Can you work these out from the model? Positions are in its coordinate system, mm. A direction names the side the tool comes from. Round coordinates to 2 decimals unless told otherwise and drop trailing zeros. Write each loop counter-clockwise with the first axis right and the second up, starting at its lowest first coordinate (ties: lowest second). Pieces come first, ordered by that corner, then holes.
Q1. Please list where these lines run through material, in increasing order: line 1 along Z through (x, y) = (-5.5, 0.4); line 2 along X through (y, z) = (1.8, 0); line 3 along Z through (x, y) = (-4, 0.9).
Q2. We'd pull the mould along X, two halves only. Please class faces 1 (the flat face through (0, 0, -1)), 2 (the cylindrical face through (26.99, 1.27, 37.15)), 3 (the flat face through (-13, 1, -20.194)): +X half, -X half, draft (parallel to the pull), parting line (faces both ways), or undercut.
Q3. If we section it at C-C (x = 0): Please give me the cut outline in (y, z).
Q4. If we section it at B-B (z = 3): Please give me the cut outline in (x, y), plus the area to 3 significant figures.
Q5. If we section it at A-A (x = 7): Please give me the cut outline in (y, z), plus the area to 3 significant figures.
Q6. For faces 4 (the flat face through (0, 1, -40)), 5 (the cylindrical face through (0.086, 1.268, -6.983)), which set-ups out of +Z, -Z, +X, -X, +Y, -Y let a thin tool reach every point of the face, with its end or its side?
Q7. If we section it at D-D (y = 0.45): Give the number of separate pieces and of enclosed holes in the cut face, plus the area to 3 significant figures.
from build123d import *

# Parameters (mm, degrees)
SKETCH_1_W          = 60
SKETCH_1_H          = 80
SKETCH_1_R          = 1.25
SKETCH_1_R_2        = 1.6
EXTRUDE_1_DEPTH     = 2.5
FILLET_1_R          = 10
CUT_EXTRUDE_1_DEPTH = 2.5
CUT_EXTRUDE_2_DEPTH = 2.5


with BuildPart() as part:
    # 草图1 → 凸台-拉伸1 (new body)
    with BuildSketch(Plane(origin=(0, 0, 0), x_dir=(1, 0, 0), z_dir=(0, 1, 0))):
        Rectangle(SKETCH_1_W, SKETCH_1_H)
        with Locations(Location((21, 33, 0), (0, 0, 270))):
            Circle(SKETCH_1_R, mode=Mode.SUBTRACT)
        with Locations(Location((-21, 33, 0), (0, 0, 90))):
            Circle(SKETCH_1_R, mode=Mode.SUBTRACT)
        with Locations(Location((-21, -33, 0), (0, 0, 270))):
            Circle(SKETCH_1_R, mode=Mode.SUBTRACT)
        with Locations(Location((21, -33, 0), (0, 0, 90))):
            Circle(SKETCH_1_R, mode=Mode.SUBTRACT)
        with Locations(Location((0, 3, 0), (0, 0, 270))):
            Circle(SKETCH_1_R_2, mode=Mode.SUBTRACT)
        with Locations(Location((3, 0, 0), (0, 0, 270))):
            Circle(SKETCH_1_R_2, mode=Mode.SUBTRACT)
        with Locations(Location((0, -3, 0), (0, 0, 90))):
            Circle(SKETCH_1_R_2, mode=Mode.SUBTRACT)
        with Locations(Location((-3, 0, 0), (0, 0, 90))):
            Circle(SKETCH_1_R_2, mode=Mode.SUBTRACT)
    extrude(amount=EXTRUDE_1_DEPTH)

    # 圆角1
    fillet_1_edges = [part.edges().sort_by_distance(p)[0] for p in [
        (30, 1.25, 40),
        (-30, 1.25, 40),
        (-30, 1.25, -40),
        (30, 1.25, -40),
    ]]
    fillet(fillet_1_edges, radius=FILLET_1_R)

    # 草图2 → 切除-拉伸1 (cut)
    with BuildSketch(Plane(origin=(0, 2.5, 0), x_dir=(1, 0, 0), z_dir=(0, 1, 0))):
        with BuildLine():
            Line((-20.730933361, 20.193862548), (20.730933361, 20.193862548))
            ThreePointArc((20.730933361, 20.193862548), (25.671984835, 15.252811074), (20.730933361, 10.311759599))
            Line((20.730933361, 10.311759599), (-20.730933361, 10.311759599))
            ThreePointArc((-20.730933361, 10.311759599), (-25.671984835, 15.252811074), (-20.730933361, 20.193862548))
        make_face()
        with BuildLine():
            Line((-20.730933361, -20.193862548), (20.730933361, -20.193862548))
            ThreePointArc((20.730933361, -20.193862548), (25.671984835, -15.252811074), (20.730933361, -10.311759599))
            Line((20.730933361, -10.311759599), (-20.730933361, -10.311759599))
            ThreePointArc((-20.730933361, -10.311759599), (-25.671984835, -15.252811074), (-20.730933361, -20.193862548))
        make_face()
    extrude(amount=-CUT_EXTRUDE_1_DEPTH, mode=Mode.SUBTRACT)

    # 草图3 → 切除-拉伸2 (cut)
    with BuildSketch(Plane(origin=(0, 2.5, 0), x_dir=(1, 0, 0), z_dir=(0, 1, 0))):
        with BuildLine():
            Line((-4.941051475, 11.922972036), (-4.941051475, 28.46475306))
            ThreePointArc((-4.941051475, 28.46475306), (0, 33.405804535), (4.941051475, 28.46475306))
            Line((4.941051475, 28.46475306), (4.941051475, 11.922972036))
            ThreePointArc((4.941051475, 11.922972036), (0, 6.981920562), (-4.941051475, 11.922972036))
        make_face()
        with BuildLine():
            Line((-4.941051475, -11.922972036), (-4.941051475, -28.46475306))
            ThreePointArc((-4.941051475, -28.46475306), (0, -33.405804535), (4.941051475, -28.46475306))
            Line((4.941051475, -28.46475306), (4.941051475, -11.922972036))
            ThreePointArc((4.941051475, -11.922972036), (0, -6.981920562), (-4.941051475, -11.922972036))
        make_face()
    extrude(amount=-CUT_EXTRUDE_2_DEPTH, mode=Mode.SUBTRACT)


solid = part.part
A:
1. line 1: z = -40 to -20.19, -10.31 to 10.31, 20.19 to 40
1. line 2: x = -30 to -4.6, -1.4 to 1.4, 4.6 to 30
1. line 3: z = -40 to -31.37, -9.02 to -1.25, 1.25 to 9.02, 31.37 to 40
2. face 1: draft
2. face 2: +X half
2. face 3: undercut
3. outline: (0, -40) - (2.5, -40) - (2.5, -33.41) - (0, -33.41) - close; (0, -6.98) - (2.5, -6.98) - (2.5, -4.6) - (0, -4.6) - close; (0, -1.4) - (2.5, -1.4) - (2.5, 1.4) - (0, 1.4) - close; (0, 4.6) - (2.5, 4.6) - (2.5, 6.98) - (0, 6.98) - close; (0, 33.41) - (2.5, 33.41) - (2.5, 40) - (0, 40) - close
4. outline: (-30, 0) - (-1.6, 0) - (-1.6, 2.5) - (-30, 2.5) - close; (1.6, 0) - (30, 0) - (30, 2.5) - (1.6, 2.5) - close
4. area: 142 mm2
5. outline: (0, -40) - (2.5, -40) - (2.5, -20.19) - (0, -20.19) - close; (0, -10.31) - (2.5, -10.31) - (2.5, 10.31) - (0, 10.31) - close; (0, 20.19) - (2.5, 20.19) - (2.5, 40) - (0, 40) - close
5. area: 151 mm2
6. face 4: -Z, +X, -X, +Y, -Y
6. face 5: +Y, -Y
7. separate pieces: 1
7. enclosed holes: 10
7. area: 3,400 mm2
